Geometry: see drawing. Coordinates: mm, zero at the bounding-box minimum. Give positions to 0.01 mm unless a question says otherwise; leave off trailing zeros. Write each loop counter-clockwise with the first axis right and the second up, starting at its lowest first coordinate (ties: lowest second). Pieces come first, ordered by that corner, then holes. Notation, with made-up numbers: (66.25, 56.25) - (99.25, 56.25) arc R16 cw to (99.25, 81.25) - close; hole circle Ø7 at (-6, 42). An arc over 180 degrees is marked (long way). Return JSON: item names as keys, results as strings.
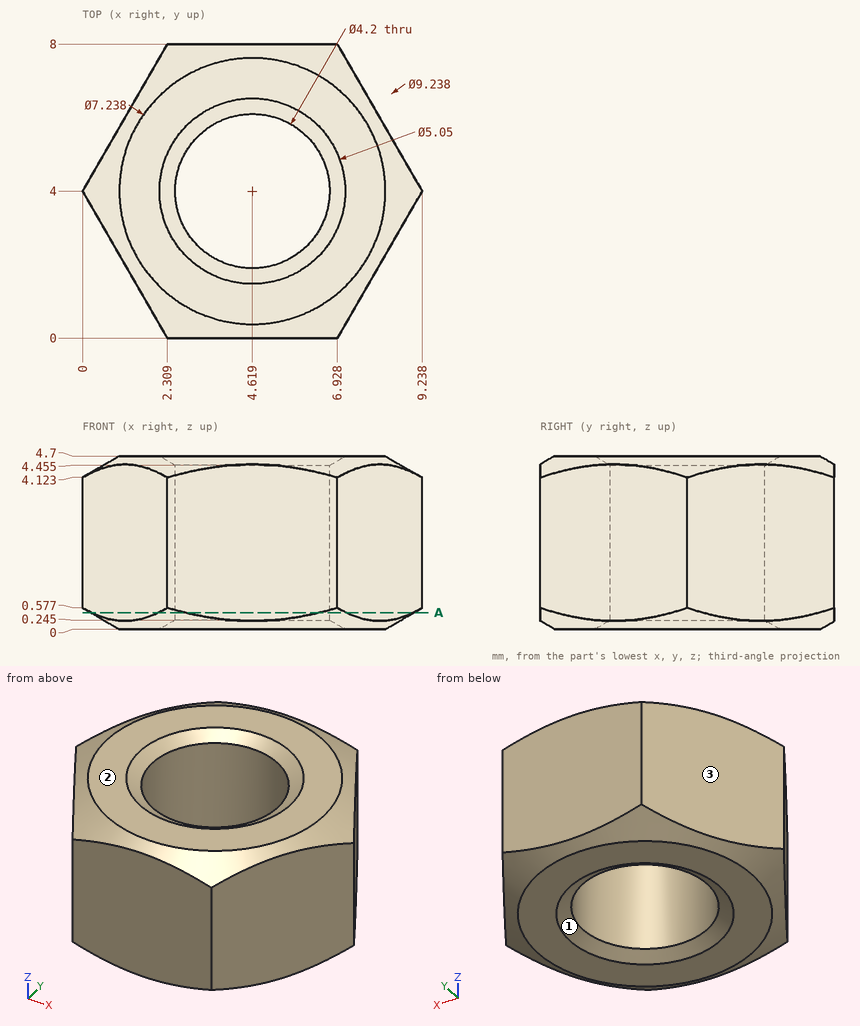
Q1. Material intervals for probe 1 along Y at (x, z) = (5.25, 3.85); probe 2 along Y at (x, z) = (4.75, 2.35) (1 decimal); probe 3 along X at (y, z) = (6.75, 3.8), sorted ascending. Write a range as [from, to].
Answer key:
{"probe 1": "y = [0, 2], [6, 8]", "probe 2": "y = [0, 1.9], [6.1, 8]", "probe 3": "x = [1.59, 7.65]"}
Q2. Section query A-A, the plane z = 0.45. Return the cut outline in (x, y).
Answer key:
{"outline": "(0.24, 3.58) - (2.07, 0.42) arc R4.4 ccw to (2.79, 0) - (6.45, 0) arc R4.4 ccw to (7.17, 0.42) - (9, 3.58) arc R4.4 ccw to (9, 4.42) - (7.17, 7.58) arc R4.4 ccw to (6.45, 8) - (2.79, 8) arc R4.4 ccw to (2.07, 7.58) - (0.24, 4.42) arc R4.4 ccw to start; hole circle Ø4.2 at (4.62, 4)"}
Q3. Mould query, pull axis X, two halves, no side actions, for the marked faces 1, 2 and 3. Classes: pulls with the +X half, pulls with the -X half, needs draft (parallel to the pull), parting line crosses it, or undercut.
Answer key:
{"face 1": "undercut", "face 2": "needs draft", "face 3": "pulls with the -X half"}
